The listing builds one solid part. Answer for the finished solid, in the listing's coordinates (mm). Round coordinates to 2 decimals unless told otherwise and drop trailing zeros. Loops run counter-clockwise (first coordinate to the right, second up) from the corner with the lowest first, then second, coordinate; pieces in that order, holes last. Notation, with made-up numbers: (-8.5, -8) -> (7.5, -8) arc R36 cw to (7.5, 29) -> close; hole circle Ø11 at (86.25, 29). An arc over 180 degrees is marked (long way). Use a Markdown table: item, result. Add a question column.
Q1. Given pin 1 Ø10 at (x, y) = (135.5, 61) entering from +Z, flat-ended and moving along its own axis, determine where the tip first touches the part or whether it passes through.
Q2. Section D-D on y = 255.5 is taken. Give the vertices of the cut face in (x, z), then the cut area to 3 significant figures.
Q3. Section C-C on x = 437.5 is taken. Give the vertices of the cut face in (y, z), then the cut area to 3 significant figures.
Q4. Consider line 1 (Y direction, x = 125.5, z = 46); line 2 (X direction, y = 32.5, z = 145); line 3 (Y direction, x = 230, z = 69.5). Determine where each line is inside the solid, lowest interval first.
Q5. Section B-B on y = 490.5 is taken. Give the vertices of the cut face in (x, z), then the cut area to 3 significant figures.
Q6. For a pull along Y with two mould halves and no side action, classify faces 1 (the flat face through (703, 349.25, 127)), 2 (the flat face through (855, 323.85, 127)), 3 (the flat face through (518, 284, 0)), 4 (the flat face through (518, 600.964, 103)) as released by +Y, released by -Y, zero draft, split by the parting line, or undercut.
Q7. Section A-A on z = 140 is taken. Give the number of separate pieces and of enclosed holes in the cut face, then the cut area to 3 significant figures.
from build123d import *

# Parameters (mm, degrees)
F0_W     = 1140.46
F0_H     = 643.128
F1_DEPTH = 209.55
F3_DEPTH = 191.77
F4_W     = 977.9
F4_H     = 495.3
F5_DEPTH = 190.5
F6_DEPTH = 25.4
F7_W     = 215.9
F7_H     = 69.85
F8_DEPTH = 165.1


with BuildPart() as f1:
    # F0 (on Top) → F1 (new body)
    with BuildSketch(Plane.XY):
        with Locations((525.78, 279.4)):
            Rectangle(F0_W, F0_H)
    extrude(amount=F1_DEPTH)

    # F2 (on face) → F3 (cut)
    with BuildSketch(Plane.XY.offset(209.55)):
        with BuildLine():
            ThreePointArc((0, 25.4), (7.4394877579, 7.4394877579), (25.4, 0))
            Line((25.4, 0), (1028.7, 0))
            ThreePointArc((1028.7, 0), (1046.6605122421, 7.4394877579), (1054.1, 25.4))
            Line((1054.1, 25.4), (1054.1, 533.4))
            ThreePointArc((1054.1, 533.4), (1046.6605122421, 551.3605122421), (1028.7, 558.8))
            Line((1028.7, 558.8), (25.4, 558.8))
            ThreePointArc((25.4, 558.8), (7.4394877579, 551.3605122421), (0, 533.4))
            Line((0, 533.4), (0, 25.4))
        make_face()
    extrude(amount=-F3_DEPTH, mode=Mode.SUBTRACT)

    # F4 (on face) → F5 (join)
    with BuildSketch(Plane.XY.offset(17.78)):
        with BuildLine():
            ThreePointArc((0, 25.4), (7.4394877579, 7.4394877579), (25.4, 0))
            Line((25.4, 0), (1028.7, 0))
            ThreePointArc((1028.7, 0), (1046.6605122421, 7.4394877579), (1054.1, 25.4))
            Line((1054.1, 25.4), (1054.1, 533.4))
            ThreePointArc((1054.1, 533.4), (1046.6605122421, 551.3605122421), (1028.7, 558.8))
            Line((1028.7, 558.8), (25.4, 558.8))
            ThreePointArc((25.4, 558.8), (7.4394877579, 551.3605122421), (0, 533.4))
            Line((0, 533.4), (0, 25.4))
        make_face()
        with Locations((527.05, 279.4)):
            Rectangle(F4_W, F4_H, mode=Mode.SUBTRACT)
    extrude(amount=F5_DEPTH)

    # F6 (add): a face of the model
    f6_faces = [f1.faces().sort_by_distance(p)[0] for p in [
        (527.05, 279.4, 17.78),
    ]]
    extrude(f6_faces, amount=F6_DEPTH)

    # F7 (on face) → F8 (join)
    with BuildSketch(Plane.XY.offset(208.28)):
        Polygon((1003.3, 31.75), (1016, 31.75), (1016, 323.85), (1016, 349.25), (381, 349.25), (381, 527.05), (355.6, 527.05), (355.6, 444.5), (273.05, 444.5), (273.05, 527.05), (247.65, 527.05), (247.65, 444.5), (114.3, 444.5), (114.3, 349.25), (38.1, 349.25), (38.1, 323.85), (38.1, 31.75), (50.8, 31.75), (50.8, 323.85), (342.9, 323.85), (342.9, 31.75), (381, 31.75), (381, 323.85), (673.1, 323.85), (673.1, 31.75), (711.2, 31.75), (711.2, 323.85), (1003.3, 323.85), align=None)
        with Locations((247.65, 384.175)):
            Rectangle(F7_W, F7_H, mode=Mode.SUBTRACT)
    extrude(amount=-F8_DEPTH)


solid = f1.part
Checked values:
| question | item | result |
|---|---|---|
| 1 | pin 1 | stops at z = 43.18 |
| 2 | outline | (-44.45, 0) -> (1096.01, 0) -> (1096.01, 209.55) -> (1054.1, 209.55) -> (1054.1, 208.28) -> (1003.3, 208.28) -> (1003.3, 43.18) -> (711.2, 43.18) -> (711.2, 208.28) -> (673.1, 208.28) -> (673.1, 43.18) -> (381, 43.18) -> (381, 208.28) -> (342.9, 208.28) -> (342.9, 43.18) -> (50.8, 43.18) -> (50.8, 208.28) -> (0, 208.28) -> (0, 209.55) -> (-44.45, 209.55) -> close |
| 2 | area | 93,000 mm2 |
| 3 | outline | (-42.16, 0) -> (600.96, 0) -> (600.96, 209.55) -> (558.8, 209.55) -> (558.8, 208.28) -> (527.05, 208.28) -> (527.05, 43.18) -> (349.25, 43.18) -> (349.25, 208.28) -> (323.85, 208.28) -> (323.85, 43.18) -> (31.75, 43.18) -> (31.75, 208.28) -> (0, 208.28) -> (0, 209.55) -> (-42.16, 209.55) -> close |
| 3 | area | 56,500 mm2 |
| 4 | line 1 | y = -42.16 to 31.75, 323.85 to 444.5, 527.05 to 600.96 |
| 4 | line 2 | x = -44.45 to 50.8, 342.9 to 381, 673.1 to 711.2, 1003.3 to 1096.01 |
| 4 | line 3 | y = -42.16 to 31.75, 323.85 to 349.25, 419.1 to 444.5, 527.05 to 600.96 |
| 5 | outline | (-44.45, 0) -> (1096.01, 0) -> (1096.01, 209.55) -> (1054.1, 209.55) -> (1054.1, 208.28) -> (1016, 208.28) -> (1016, 43.18) -> (381, 43.18) -> (381, 208.28) -> (355.6, 208.28) -> (355.6, 43.18) -> (273.05, 43.18) -> (273.05, 208.28) -> (247.65, 208.28) -> (247.65, 43.18) -> (38.1, 43.18) -> (38.1, 208.28) -> (0, 208.28) -> (0, 209.55) -> (-44.45, 209.55) -> close |
| 5 | area | 84,600 mm2 |
| 6 | face 1 | undercut |
| 6 | face 2 | undercut |
| 6 | face 3 | zero draft |
| 6 | face 4 | released by +Y |
| 7 | separate pieces | 1 |
| 7 | enclosed holes | 7 |
| 7 | area | 318,000 mm2 |
